Autodesk Inventor part; units mm, degrees
ref_plane "YZ Plane" through (0, 0, 0) normal (1, 0, 0) x (0, 1, 0)
ref_plane "XZ Plane" through (0, 0, 0) normal (0, 1, 0) x (-1, 0, 0)
ref_plane "XY Plane" through (0, 0, 0) normal (0, 0, 1) x (1, 0, 0)
sketch "Sketch1" plane through (0, 0, 0) normal (0, 1, 0) x (-1, 0, 0)
  circle A0 centre (-18, -24.5) radius 13 construction
  circle A1 centre (-140.57, -24.5) radius 13 construction
  circle A2 centre (-4.1, -24.5) radius 0.9 construction
  circle A3 centre (-154.47, -24.5) radius 0.9 construction
  line L0 (0, -42.5) -> (-158.57, -42.5)
  line L1 (-158.57, -42.5) -> (-158.57, -6.5)
  line L2 (0, -6.5) -> (0, -42.5)
  line L3 (-22, -6.5) -> (-22, 0)
  line L4 (-22, 0) -> (-136.57, 0)
  line L5 (-136.57, 0) -> (-136.57, -6.5)
  line L6 (-158.57, -6.5) -> (-136.57, -6.5)
  line L7 (-22, -6.5) -> (0, -6.5)
  circle A4 centre (-18, -24.5) radius 17 construction
  circle A5 centre (-18, -24.5) radius 4.25
  circle A6 centre (-140.57, -24.5) radius 4.25
  point P0 (0, 0)
  point P1 (0, -24.5)
  dimension "d0" = 26
  dimension "d1" = 1.8
  dimension "d3" = 150.37
  dimension "d4" = 36
  dimension "d5" = 18
  dimension "d6" = 18
  dimension "d7" = 6.5
  dimension "d8" = 34
  dimension "d9" = 22
  dimension "d10" = 22
  dimension "d11" = 8.5
extrude "Extrusion1" add sketch "Sketch1" along normal blind 6.5
chamfer "Chamfer1" distance 10 angle 45 4 edges at (0, 3.25, -42.5) (0, 3.25, -6.5) (158.57, 3.25, -6.5) (158.57, 3.25, -42.5)
sketch "Sketch2" plane through (0, 6.5, 0) normal (0, 1, 0) x (1, 0, 0)
  line L0 (148.57, 42.5) -> (10, 42.5)
  line L1 (158.57, 16.5) -> (148.57, 6.5)
  line L2 (158.57, 16.5) -> (158.57, 32.5)
  line L3 (26, 42.5) -> (36, 32.5)
  line L4 (36, 32.5) -> (122.57, 32.5)
  line L5 (122.57, 32.5) -> (132.57, 42.5)
  line L6 (26, 42.5) -> (132.57, 42.5)
  point P0 (0, 32.5)
  point P1 (0, 16.5)
  point P2 (0, 0)
  dimension "d17" = 10
  dimension "d18" = 16
  dimension "d19" = 16
  dimension "d20" = 16
extrude "Extrusion2" cut sketch "Sketch2" against normal through all
sketch "Sketch3" plane through (0, 6.5, 0) normal (0, 1, 0) x (1, 0, 0)
  line L0 (22, 0) -> (136.57, 0)
  circle A0 centre (140.57, 24.5) radius 4.25
  circle A1 centre (18, 24.5) radius 4.25
  line L1 (36.57, 16.5) -> (121.57, 16.5) construction
  line L2 (121.57, 16.5) -> (121.57, 10) construction
  line L3 (121.57, 10) -> (36.57, 10) construction
  line L4 (36.57, 10) -> (36.57, 16.5) construction
  circle A2 centre (18, 24.5) radius 17 construction
  circle A3 centre (140.57, 24.5) radius 17 construction
  line L5 (42.57, 16.5) -> (50.57, 16.5)
  line L6 (50.57, 16.5) -> (50.57, 10)
  line L7 (50.57, 10) -> (42.57, 10)
  line L8 (42.57, 10) -> (42.57, 16.5)
  line L9 (75.07, 16.5) -> (83.07, 16.5)
  line L10 (83.07, 16.5) -> (83.07, 10)
  line L11 (83.07, 10) -> (75.07, 10)
  line L12 (75.07, 10) -> (75.07, 16.5)
  line L13 (107.57, 16.5) -> (115.57, 16.5)
  line L14 (115.57, 16.5) -> (115.57, 10)
  line L15 (115.57, 10) -> (107.57, 10)
  line L16 (107.57, 10) -> (107.57, 16.5)
  line L17 (50.57, 13.25) -> (75.07, 13.25) construction
  line L18 (83.07, 13.25) -> (107.57, 13.25) construction
  point P0 (0, 0)
  dimension "d23" = 6.5
  dimension "d24" = 85
  dimension "d25" = 34
  dimension "d26" = 34
  dimension "d27" = 19
  dimension "d28" = 10
  dimension "d29" = 8
  dimension "d30" = 6
  dimension "d31" = 6
extrude "Extrusion3" cut sketch "Sketch3" against normal through all contours L5 L6 L7 L8 | L9 L10 L11 L12 | L13 L14 L15 L16
chamfer "Chamfer2" distance 2 angle 45 2 edges at (22, 3.25, -6.5) (136.57, 3.25, -6.5)
sketch "Sketch4" plane through (0, 6.5, 0) normal (0, 1, 0) x (1, 0, 0)
  line L0 (22, 0) -> (136.57, 0)
  line L1 (136.57, 0) -> (136.57, 4.5)
  line L2 (132.57, 0) -> (124.57, 0)
  line L3 (124.57, 0) -> (124.57, -4.5)
  line L4 (126.57, -6.5) -> (130.57, -6.5)
  line L5 (132.57, -4.5) -> (132.57, 0)
  line L6 (82.57, 0) -> (74.57, 0)
  line L7 (74.57, 0) -> (74.57, -4.5)
  line L8 (76.57, -6.5) -> (80.57, -6.5)
  line L9 (82.57, -4.5) -> (82.57, 0)
  line L10 (42.57, 0) -> (34.57, 0)
  line L11 (34.57, 0) -> (34.57, -4.5)
  line L12 (36.57, -6.5) -> (40.57, -6.5)
  line L13 (42.57, -4.5) -> (42.57, 0)
  arc A0 (124.57, -4.5) -> (126.57, -6.5) centre (126.57, -4.5) ccw
  arc A1 (130.57, -6.5) -> (132.57, -4.5) centre (130.57, -4.5) ccw
  arc A2 (80.57, -6.5) -> (82.57, -4.5) centre (80.57, -4.5) ccw
  arc A3 (74.57, -4.5) -> (76.57, -6.5) centre (76.57, -4.5) ccw
  arc A4 (40.57, -6.5) -> (42.57, -4.5) centre (40.57, -4.5) ccw
  arc A5 (34.57, -4.5) -> (36.57, -6.5) centre (36.57, -4.5) ccw
  point P0 (0, 0)
  dimension "d37" = 2
  dimension "d38" = 8
  dimension "d39" = 8
  dimension "d40" = 8
  dimension "d41" = 6.5
  dimension "d42" = 4
  dimension "d43" = 42
  dimension "d44" = 82
extrude "Extrusion4" add sketch "Sketch4" against normal blind 6.5
equation "\"d5\" = 0.5 * d4"
equation "\"d6\" = d5"
equation "\"d10\" = d9"
equation "\"d19\" = d18"
equation "\"d20\" = d19"
equation "\"d31\" = d30"
equation "\"d39\" = d38"
equation "\"d40\" = d39"
properties part number "z_pulley_holder_right" material "Plywood, Finish"
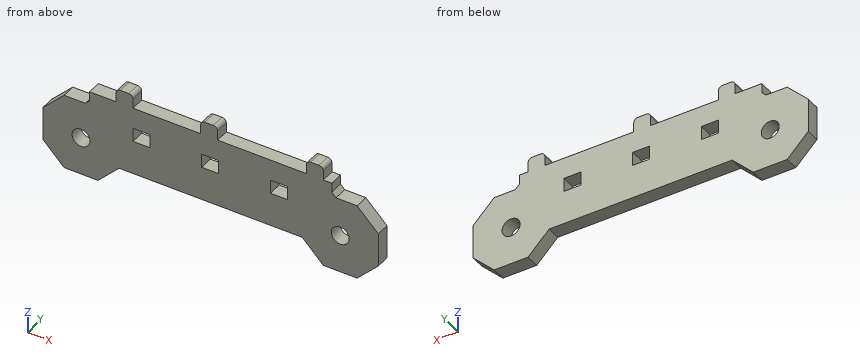
Geometry check sheet. Reference: the model listing, model coordinates, mm. Coordinates: 2 decimals unless noted, no trailing zeros. Loops run counter-clockwise (first coordinate to the right, second up) from the corner with the lowest first, then second, coordinate; pieces in that order, holes last. Notation, with made-up numbers: (33.25, 49.5) - (45.25, 49.5) arc R24 cw to (45.25, 60.5) - close; hole circle Ø4 at (42, 17). An arc over 180 degrees is marked (long way). One line per item, written item: value. Start each with the question number.
(1) Material ranges on line 1 (X direction, y = 1, z = 3); line 2 (Z direction, x = 18, y = 4); line 3 (Z direction, x = 134.5, y = 4), recorded low to high. Write a range as [from, to].
(2) Cross-section at A-A on x = 140.57. Enter the section's corners in (y, z).
(3) Cross-section at D-D on y = 2.75. Count the separate pieces of the cut face and the enclosed holes in it, plus the area to 3 significant figures.
(4) Depth check by flat-ended pin: P1, Ø3, axis at y = 3.5, z = -12, coming from the -X side; P2, Ø3, axis at y = 2.5, z = -12.5, coming from the +X side; P3, Ø1, axis at y = 4, z = -1.5, coming from the +X side; P4, Ø1, axis at x = 107, z = -2, coming from the -Y side. Enter the tip coordinate at first touch or a pass-through.
(5) Cross-section at C-C on z = -34. Enter the section's corners in (x, y).
(6) Cross-section at B-B on z = -24.5. Enter the section's corners in (x, y).
Results below:
1. line 1: x = [34.57, 42.57], [74.57, 82.57], [124.57, 132.57]
1. line 2: z = [-42.5, -28.75], [-20.25, -6.5]
1. line 3: z = [-42.5, 0]
2. outline: (0, -42.5) - (6.5, -42.5) - (6.5, -28.75) - (0, -28.75) - close; (0, -20.25) - (6.5, -20.25) - (6.5, -6.5) - (0, -6.5) - close
3. separate pieces: 1
3. enclosed holes: 5
3. area: 5,170 mm2
4. P1: stops at x = 3
4. P2: stops at x = 156.07
4. P3: stops at x = 136.57
4. P4: stops at y = 0
5. outline: (1.5, 0) - (34.5, 0) - (34.5, 6.5) - (1.5, 6.5) - close; (124.07, 0) - (157.07, 0) - (157.07, 6.5) - (124.07, 6.5) - close
6. outline: (0, 0) - (13.75, 0) - (13.75, 6.5) - (0, 6.5) - close; (22.25, 0) - (136.32, 0) - (136.32, 6.5) - (22.25, 6.5) - close; (144.82, 0) - (158.57, 0) - (158.57, 6.5) - (144.82, 6.5) - close
